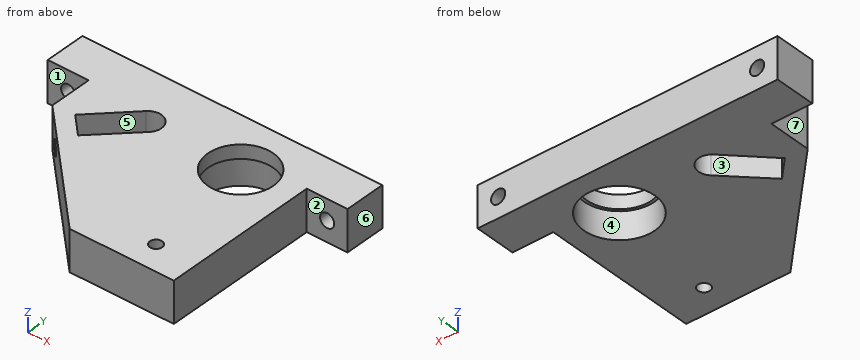
```python
from build123d import *

# Parameters (mm, degrees)
SKETCH_1_R          = 12
SKETCH_1_R_2        = 2.25
EXTRUDE_1_DEPTH     = 15
SKETCH_2_R          = 13
CUT_EXTRUDE_1_DEPTH = 10
SKETCH_3_R          = 2.6
CUT_EXTRUDE_2_DEPTH = 73.5
SKETCH_5_R          = 2.6
CUT_EXTRUDE_3_DEPTH = 10


with BuildPart() as part:
    # 草图1 → 凸台-拉伸1 (new body)
    with BuildSketch(Plane.XY):
        Polygon((-33.800989673, 26.429197467), (-27.44059998, 26.429197467), (-18.800989673, 26.429197467), (-18.800989673, 10.718519348), (22.988332208, -31.070802533), (61.199010327, -31.070802533), (61.199010327, 26.429197467), (76.199010327, 26.429197467), (76.199010327, 41.429197467), (56.199010327, 41.429197467), (-33.800989673, 41.429197467), align=None)
        with Locations((41.199010327, 21.429197467)):
            Circle(SKETCH_1_R, mode=Mode.SUBTRACT)
        with Locations((46.199010327, -21.070802533)):
            Circle(SKETCH_1_R_2, mode=Mode.SUBTRACT)
        with BuildLine():
            Line((-11.034973369, 11.437784418), (2.9923212, 25.648765615))
            ThreePointArc((2.9923212, 25.648765615), (10.086164278, 25.671985824), (10.063536665, 18.57814083))
            Line((10.063536665, 18.57814083), (-4.055896558, 4.458707607))
            Line((-4.055896558, 4.458707607), (-11.034973369, 11.437784418))
        make_face(mode=Mode.SUBTRACT)
    extrude(amount=EXTRUDE_1_DEPTH)

    # 草图2 → 切除-拉伸1 (cut)
    with BuildSketch(Plane(origin=(0, 0, 0), x_dir=(-1, 0, 0), z_dir=(0, 0, -1))):
        with Locations((-41.199010327, 21.429197467)):
            Circle(SKETCH_2_R)
    extrude(amount=-CUT_EXTRUDE_1_DEPTH, mode=Mode.SUBTRACT)

    # 草图3 → 切除-拉伸2 (cut, through all)
    with BuildSketch(Plane(origin=(0, 41.429197467, 0), x_dir=(1, 0, 0), z_dir=(0, 1, 0))):
        with Locations((-26.300989673, -7.5)):
            Circle(SKETCH_3_R)
        with Locations((68.699010327, -7.5)):
            Circle(SKETCH_3_R)
    extrude(amount=-CUT_EXTRUDE_2_DEPTH, mode=Mode.SUBTRACT)

    # 草图5 → 切除-拉伸3 (cut)
    with BuildSketch(Plane(origin=(-4.041235162, -4.041235162, 0), x_dir=(0, 0, 1), z_dir=(-0.707106781, -0.707106781, 0))):
        with Locations((7.5, 11.023445006)):
            Circle(SKETCH_5_R)
    extrude(amount=-CUT_EXTRUDE_3_DEPTH, mode=Mode.SUBTRACT)


solid = part.part
```
Design review of the part built by this model. Coordinates are the model's own, in mm. Face numbers are marked on the shaded views. A direction names the side the tool comes from. Coordinates: 2 decimals unless noted, no trailing zeros. Loops run counter-clockwise (first coordinate to the right, second up) from the corner with the lowest first, then second, coordinate; pieces in that order, holes last.
Q1. We need section D-D on y = 13.5. State the section outline as (x, z) points.
Reported:
outline: (-18.8, 0) - (-9, 0) - (-9, 15) - (-18.8, 15) - close; (4.99, 0) - (30.9, 0) - (30.9, 10) - (32.19, 10) - (32.19, 15) - (4.99, 15) - close; (50.21, 10) - (51.5, 10) - (51.5, 0) - (61.2, 0) - (61.2, 15) - (50.21, 15) - close
Q2. The part is to be moulded in two halves that separate along X. For the marked faces 5, 6 and 7, say which applies: +X half, -X half, draft (parallel to the pull), parting line (faces both ways), or undercut.
Reported:
face 5: undercut
face 6: +X half
face 7: -X half
Q3. For pin 1 (6 mm diameter, centred on y = 18.5, z = 2, fed in from +X); pin 2 (1 mm diameter, centred on x = 17.5, z = 11, fed in from -Y); pin 3 (7 mm diameter, centred on x = -26.3, z = 7.5, fed in from -Y), all flat-tipped, find the tip position at first contact; note any pin that passes through.
Reported:
pin 1: stops at x = 61.2
pin 2: stops at y = -26.08
pin 3: stops at y = 26.43
Q4. To check wall thickness, follow line 1 (Y direction, x = 41, z = 13.75); line 2 (Y direction, x = 42, z = 8.5); line 3 (X direction, y = 22.5, z = 2.5). State the ranges of each line that lie inside material, in increasing order.
Reported:
line 1: y = -31.07 to 9.43, 33.43 to 41.43
line 2: y = -31.07 to 8.45, 34.4 to 41.43
line 3: x = -18.8 to -0.12, 11.54 to 28.24, 54.15 to 61.2
Q5. We need section A-A on y = 28.5. State the section outline as (x, z) points.
Reported:
outline: (-33.8, 0) - (30.29, 0) - (30.29, 10) - (31.5, 10) - (31.5, 15) - (-33.8, 15) - close; (50.89, 10) - (52.11, 10) - (52.11, 0) - (76.2, 0) - (76.2, 15) - (50.89, 15) - close; hole circle Ø5.2 at (-26.3, 7.5); hole circle Ø5.2 at (68.7, 7.5)
Q6. Tool access review of the marked faces 1, 2, 3 and 4: name each direction out of +Z, -Z, +X, -X, +Y, -Y from which nothing blocks a thin tool from reaching the whole face with its end or side.
Reported:
face 1: +Z, -Z, -X, -Y
face 2: +Z, -Z, +X, -Y
face 3: +Z, -Z
face 4: -Z
Q7. We need section B-B on x = 52. State the section outline as (y, z) points, and give its area (3 significant figures).
Reported:
outline: (-31.07, 0) - (14.19, 0) - (14.19, 10) - (16.2, 10) - (16.2, 15) - (-31.07, 15) - close; (26.66, 10) - (28.66, 10) - (28.66, 0) - (41.43, 0) - (41.43, 15) - (26.66, 15) - close
area: 891 mm2
Q8. We need section C-C on z = 7.5. State the section outline as (x, y) points.
Reported:
outline: (-33.8, 26.43) - (-28.9, 26.43) - (-28.9, 41.43) - (-33.8, 41.43) - close; (-23.7, 26.43) - (-18.8, 26.43) - (-18.8, 10.72) - (-13.67, 5.59) - (-9.43, 9.83) - (-11.03, 11.44) - (2.99, 25.65) arc R5 cw (long way) to (10.06, 18.58) - (-4.06, 4.46) - (-5.75, 6.16) - (-10, 1.92) - (22.99, -31.07) - (61.2, -31.07) - (61.2, 26.43) - (66.1, 26.43) - (66.1, 41.43) - (-23.7, 41.43) - close; (71.3, 26.43) - (76.2, 26.43) - (76.2, 41.43) - (71.3, 41.43) - close; hole circle Ø26 at (41.2, 21.43); hole circle Ø4.5 at (46.2, -21.07)
